For this review, take the finished solid that the model builds, in its own axes (mm). Face numbers are marked on the shaded views. A direction names the side the tool comes from. Round coordinates to 2 decimals unless told otherwise and drop trailing zeros. Order: outer loops, then holes, each group sorted by start corner. A loop starts at its lowest first (then second) coordinate and runs counter-clockwise, first axis right, second up.
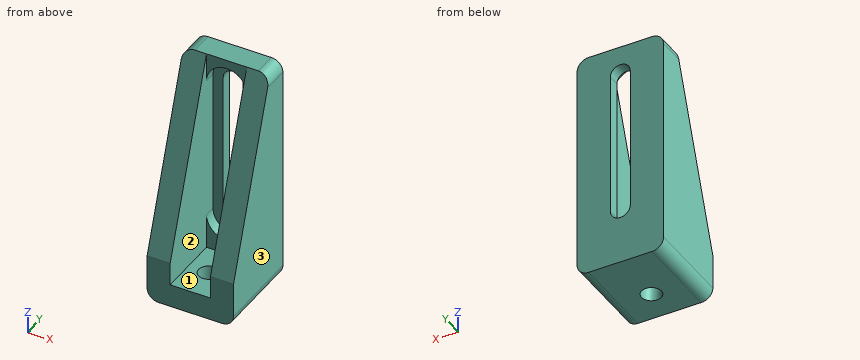
```python
from build123d import *

# Parameters (mm, degrees)
F0_W     = 15
F0_H     = 15.2
F0_R     = 1.725
F1_DEPTH = 4
F3_DEPTH = 36
F5_DEPTH = 2
F6_DEPTH = 4
F7_SIZE2 = 11.2
F7_SIZE  = 32
F8_R     = 2


with BuildPart() as f1:
    # F0 (on Top) → F1 (new body)
    with BuildSketch(Plane.XY):
        Rectangle(F0_W, F0_H)
        with Locations((0, -2)):
            Circle(F0_R, mode=Mode.SUBTRACT)
    extrude(amount=F1_DEPTH)

    # F2 (on face) → F3 (join)
    with BuildSketch(Plane.XY.offset(4)):
        Polygon((-7.5, 7.6), (-7.5, -7.6), (-3.5, -7.6), (-3.5, -2), (-3.5, 3.6), (3.5, 3.6), (3.5, -2), (3.5, -7.6), (7.5, -7.6), (7.5, 7.6), align=None)
    extrude(amount=F3_DEPTH)

    # F4 (on face) → F5 (cut)
    with BuildSketch(Plane.XZ.offset(-3.6)):
        with BuildLine():
            Line((-1.725, 13.045385854), (-1.725, 31.954614146))
            ThreePointArc((-1.725, 31.954614146), (-3.0238634228, 33.2375443268), (-3.5, 35))
            Line((-3.5, 35), (-3.5, 10))
            ThreePointArc((-3.5, 10), (-3.0238634228, 11.7624556732), (-1.725, 13.045385854))
        make_face()
        with BuildLine():
            ThreePointArc((3.5, 35), (3.0238634228, 33.2375443268), (1.725, 31.954614146))
            Line((1.725, 31.954614146), (1.725, 13.045385854))
            ThreePointArc((1.725, 13.045385854), (3.0238634228, 11.7624556732), (3.5, 10))
            Line((3.5, 10), (3.5, 35))
        make_face()
        with BuildLine():
            ThreePointArc((-1.725, 35), (0, 36.725), (1.725, 35))
            Line((1.725, 35), (1.725, 31.954614146))
            ThreePointArc((1.725, 31.954614146), (3.0238634228, 33.2375443268), (3.5, 35))
            ThreePointArc((3.5, 35), (0, 38.5), (-3.5, 35))
            ThreePointArc((-3.5, 35), (-3.0238634228, 33.2375443268), (-1.725, 31.954614146))
            Line((-1.725, 31.954614146), (-1.725, 35))
        make_face()
        with BuildLine():
            ThreePointArc((3.5, 10), (3.0238634228, 11.7624556732), (1.725, 13.045385854))
            Line((1.725, 13.045385854), (1.725, 10))
            ThreePointArc((1.725, 10), (0, 8.275), (-1.725, 10))
            Line((-1.725, 10), (-1.725, 13.045385854))
            ThreePointArc((-1.725, 13.045385854), (-3.0238634228, 11.7624556732), (-3.5, 10))
            ThreePointArc((-3.5, 10), (0, 6.5), (3.5, 10))
        make_face()
    extrude(amount=-F5_DEPTH, mode=Mode.SUBTRACT)

    # F4 (on face) → F6 (cut, through all)
    with BuildSketch(Plane.XZ.offset(-3.6)):
        with BuildLine():
            ThreePointArc((-1.725, 35), (0, 33.275), (1.725, 35))
            ThreePointArc((1.725, 35), (0, 36.725), (-1.725, 35))
        make_face()
        with BuildLine():
            Line((1.725, 31.954614146), (1.725, 35))
            ThreePointArc((1.725, 35), (0, 33.275), (-1.725, 35))
            Line((-1.725, 35), (-1.725, 31.954614146))
            ThreePointArc((-1.725, 31.954614146), (0, 31.5), (1.725, 31.954614146))
        make_face()
        with BuildLine():
            Line((1.725, 13.045385854), (1.725, 31.954614146))
            ThreePointArc((1.725, 31.954614146), (0, 31.5), (-1.725, 31.954614146))
            Line((-1.725, 31.954614146), (-1.725, 13.045385854))
            ThreePointArc((-1.725, 13.045385854), (0, 13.5), (1.725, 13.045385854))
        make_face()
        with BuildLine():
            Line((1.725, 10), (1.725, 13.045385854))
            ThreePointArc((1.725, 13.045385854), (0, 13.5), (-1.725, 13.045385854))
            Line((-1.725, 13.045385854), (-1.725, 10))
            ThreePointArc((-1.725, 10), (0, 11.725), (1.725, 10))
        make_face()
        with BuildLine():
            ThreePointArc((-1.725, 10), (0, 8.275), (1.725, 10))
            ThreePointArc((1.725, 10), (0, 11.725), (-1.725, 10))
        make_face()
    extrude(amount=-F6_DEPTH, mode=Mode.SUBTRACT)

    # F7
    f7_edges = [f1.edges().sort_by_distance(p)[0] for p in [
        (5.5, -7.6, 40),
        (-5.5, -7.6, 40),
    ]]
    f7_side = f1.faces().sort_by_distance((-7.0728, -7.6, 20))[0]
    chamfer(f7_edges, length=F7_SIZE, length2=F7_SIZE2, reference=f7_side)

    # F8
    f8_edges = [f1.edges().sort_by_distance(p)[0] for p in [
        (-7.5, 5.6, 40),
        (7.5, 5.6, 40),
        (-7.5, 0, 0),
        (7.5, 0, 0),
    ]]
    fillet(f8_edges, radius=F8_R)


solid = f1.part
```
Q1. Tool access review of the marked faces 1, 2 and 3: name each direction out of +Z, -Z, +X, -X, +Y, -Y from which nothing blocks a thin tool from reaching the whole face with its end or side.
Q2. Wall thickness on line 1 (X direction, y = 6, z = 34) (3 decimals); line 2 (X direction, y = 4, z = 11); line 3 (Y direction, x = 0, z = 2.15) (3 decimals): over which ranges is each line inside the solid? List them lowest first.
Q3. Take a section at C-C, the plane y = -5.5. State the section outline as (x, z) points.
Q4. Clearance check with flat-ended pins moving along their axes: pin 1 (1.5 mm diameter, centred on x = 1.5, z = 37.5, fed in from -Y); pin 2 (2 mm diameter, centred on x = -1, y = -5, fed in from +Z); pin 3 (5.5 mm diameter, centred on x = 1, z = 23, fed in from -Y). State where each tip first meets the part, or that it passes through.
Q5. Take a section at A-A, the plane y = -2. State the section outline as (x, z) points (3 decimals).
Q6. Take a section at D-D, the plane y = 4.25. State the section outline as (x, z) points.
Q7. Take a section at B-B, the plane x = 0. State the section outline as (y, z) points (3 decimals), plus the area to 3 significant figures.
Working result:
1. face 1: +Z, -Y
1. face 2: -Y
1. face 3: +Z, -Z, +X, +Y, -Y
2. line 1: x = -7.5 to -1.725, 1.725 to 7.5
2. line 2: x = -7.5 to -3.5, 3.5 to 7.5
2. line 3: y = -7.6 to -3.725, -0.275 to 7.6
3. outline: (-7.5, 2) arc R2 ccw to (-5.5, 0) - (5.5, 0) arc R2 ccw to (7.5, 2) - (7.5, 14) - (3.5, 14) - (3.5, 4) - (-3.5, 4) - (-3.5, 14) - (-7.5, 14) - close
4. pin 1: stops at y = 3.6
4. pin 2: stops at z = 4
4. pin 3: stops at y = -2.75
5. outline: (-7.5, 2) arc R2 ccw to (-5.5, 0) - (-1.725, 0) - (-1.725, 4) - (-3.5, 4) - (-3.5, 24) - (-7.5, 24) - close; (1.725, 0) - (5.5, 0) arc R2 ccw to (7.5, 2) - (7.5, 24) - (3.5, 24) - (3.5, 4) - (1.725, 4) - close
6. outline: (-7.5, 2) arc R2 ccw to (-5.5, 0) - (5.5, 0) arc R2 ccw to (7.5, 2) - (7.5, 38) arc R2 ccw to (5.5, 40) - (-5.5, 40) arc R2 ccw to (-7.5, 38) - close; hole (-3.5, 10) arc R3.5 ccw to (3.5, 10) - (3.5, 35) arc R3.5 ccw to (-3.5, 35) - close
7. outline: (-7.6, 0) - (-3.725, 0) - (-3.725, 4) - (-7.6, 4) - close; (-0.275, 0) - (7.6, 0) - (7.6, 8.275) - (5.6, 8.275) - (5.6, 6.5) - (3.6, 6.5) - (3.6, 4) - (-0.275, 4) - close; (3.6, 38.5) - (5.6, 38.5) - (5.6, 36.725) - (7.6, 36.725) - (7.6, 40) - (3.6, 40) - close
7. area: 70.1 mm2
